Verification items for the finished model (mm, model axes). Coordinates: 2 decimals unless noted, no trailing zeros. Order: outer loops, then holes, each group sorted by start corner. A loop starts at its lowest first (then second) coordinate and runs counter-clockwise, first axis right, second up.
Q1. Cross-section at C-C, the plane y = -6.5. Record the boundary of the cut face in (x, z).
Q2. Depth check by flat-ended pin: P1, Ø4, axis at x = -147.5, y = -5, coming from the -Z side; P2, Ø1, axis at y = -14, z = -106.5, coming from the +X side; P3, Ø10, axis at y = -4.5, z = 22, coming from the +X side. Enter the tip coordinate at first touch or a pass-through.
Q3. Thickness scan on line 1 (X direction, y = -3, z = 55); line 2 (X direction, y = -2, z = -229); line 3 (Z direction, x = -65, y = -10.25). Record the ranges inside material, lowest first.
from build123d import *

# Parameters (mm, degrees)
F1_DEPTH = 19.05
F2_SIZE2 = 9.765156
F2_SIZE  = 19.04999
F3_SIZE2 = 19.04999
F3_SIZE  = 19.04999


# Not quite as in the source:
# - a fillet or chamfer is up to 0.001 mm smaller than in the source, because OpenCascade refuses the exact size


with BuildPart() as f1:
    # F0 (on Front) → F1 (new body)
    with BuildSketch(Plane.XZ):
        Polygon((-205.980393503, 296.4747510433), (-205.980393503, -389.3252489567), (98.819606497, -389.3252489567), align=None)
    extrude(amount=F1_DEPTH)

    # F2 (size 19.05 and 9.7651655461 in the source; OpenCascade refuses exactly that, so slightly less here)
    f2_edges = [f1.edges().sort_by_distance(p)[0] for p in [
        (-53.580394, 0, -389.325249),
    ]]
    f2_side = f1.faces().sort_by_distance((-53.580394, -9.525, -389.325249))[0]
    chamfer(f2_edges, length=F2_SIZE, length2=F2_SIZE2, reference=f2_side)

    # F3 (size 19.05 and 19.05 in the source; OpenCascade refuses exactly that, so slightly less here)
    f3_edges = [f1.edges().sort_by_distance(p)[0] for p in [
        (-53.580394, -19.05, -46.425249),
    ]]
    chamfer(f3_edges, length=F3_SIZE, length2=F3_SIZE2)


solid = f1.part
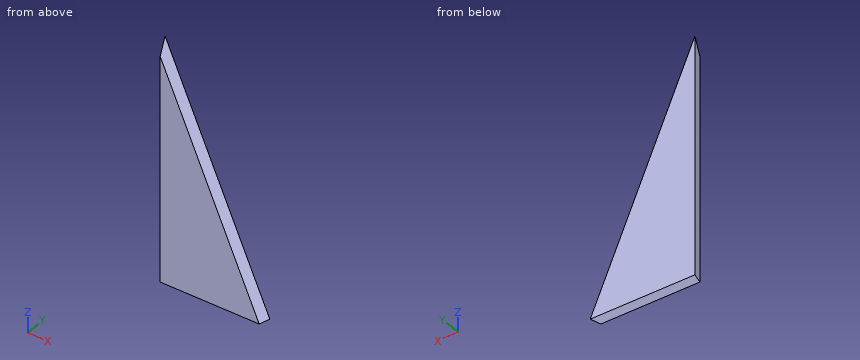
Check values:
1. outline: (-205.98, -382.89) - (88.85, -382.89) - (-205.98, 280.47) - close
2. P1: stops at z = -383.15
2. P2: stops at x = -41.61
2. P3: stops at x = -83.02
3. line 1: x = -205.98 to -101.94
3. line 2: x = -205.98 to 25.38
3. line 3: z = -384.81 to -45.97
